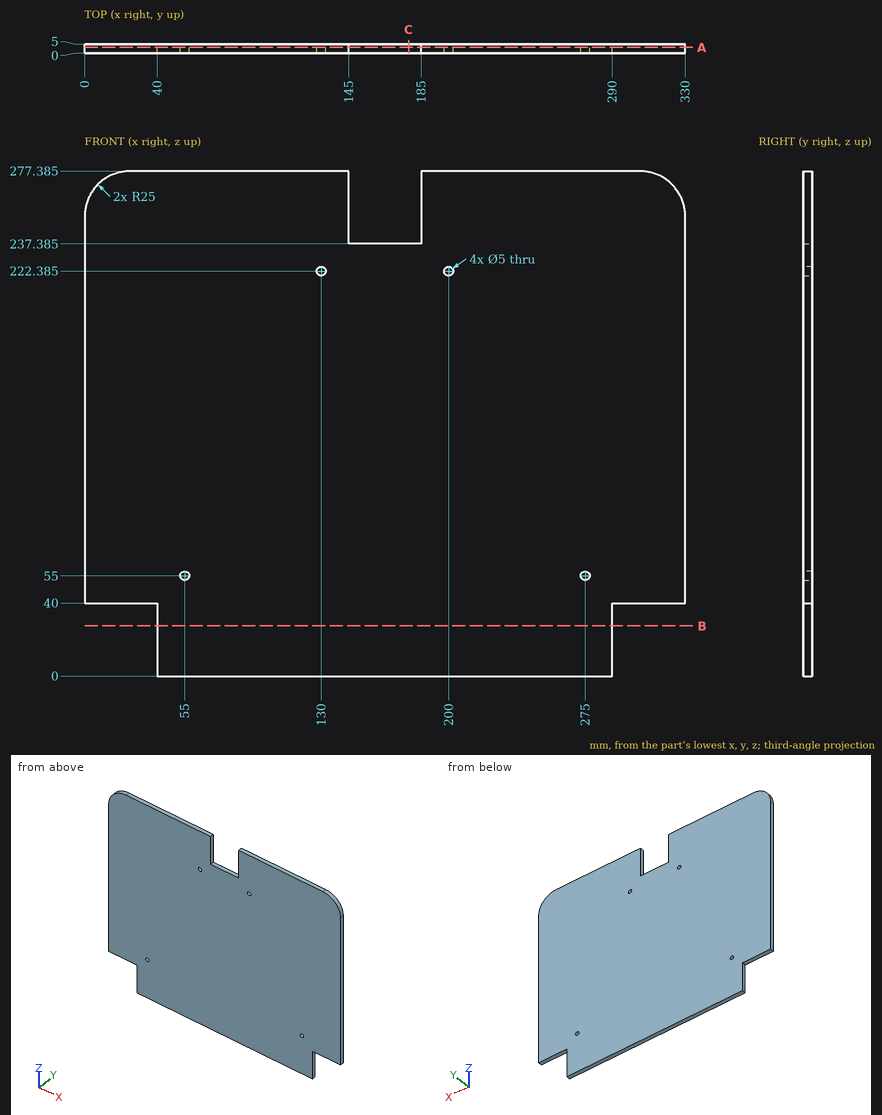
Input: dimensioned drawing with shaded views. Units: mm. Origin: part minimum x, y, z. Coordinates: 2 decimals unless noted, no trailing zeros. Loops run counter-clockwise (first coordinate to the right, second up) from the corner with the lowest first, then second, coordinate; pieces in that order, holes last. Notation, with made-up numbers: (79, -3.75) -> (83, -3.75) arc R15 ccw to (83, 9.25) -> close; hole circle Ø1 at (85, 83.5). An arc over 180 degrees is marked (long way). One line per item, written item: value. Start each with the question number.
Q1. Section query B-B, the plane z = 27.5. Return the cut outline in (x, y), and give its area (3 significant figures).
Q2. Section query A-A, the plane y = 3.2. Return the cut outline in (x, z) (1 decimal), and give its area (3 significant figures).
Q3. Section query C-C, the plane x = 178. Return the cut outline in (y, z) (1 decimal), and give its area (3 significant figures).
Q4. Contact query for flat-ended pins moving along their axis: P1, Ø1.5, axis at x = 311.5, y = 2.5, coming from the -Z side; P2, Ø2.5, axis at x = 171, y = 2, coming from the +Z side (3 decimals); P3, Ø2.5, axis at y = 3.5, z = 22, coming from the -X side. Output: stop coordinate, or through.
Q5. Line query: line 1 along X through (y, z) = (2.6, 245); line 2 along X through (y, z) = (1.2, 55); line 3 along Z through (x, y) = (200, 2.9) (1 decimal). Output: solid intervals per line, ascending.
Results:
1. outline: (40, 0) -> (290, 0) -> (290, 5) -> (40, 5) -> close
1. area: 1,250 mm^2
2. outline: (0, 40) -> (40, 40) -> (40, 0) -> (290, 0) -> (290, 40) -> (330, 40) -> (330, 252.4) arc R25 ccw to (305, 277.4) -> (185, 277.4) -> (185, 237.4) -> (145, 237.4) -> (145, 277.4) -> (25, 277.4) arc R25 ccw to (0, 252.4) -> close; hole circle Ø5 at (55, 55); hole circle Ø5 at (130, 222.4); hole circle Ø5 at (200, 222.4); hole circle Ø5 at (275, 55)
2. area: 86,400 mm^2
3. outline: (0, 0) -> (5, 0) -> (5, 237.4) -> (0, 237.4) -> close
3. area: 1,190 mm^2
4. P1: z = 40
4. P2: z = 237.385
4. P3: x = 40
5. line 1: 0 to 145, 185 to 330
5. line 2: 0 to 52.5, 57.5 to 272.5, 277.5 to 330
5. line 3: 0 to 219.9, 224.9 to 277.4
